```python
from build123d import *

# Parameters (mm, degrees)
BOSS_EXTRUDE1_DEPTH = 88.9
SKETCH2_R           = 3.175
CUT_EXTRUDE1_DEPTH  = 38.1
SKETCH3_R           = 4.1275
CUT_EXTRUDE2_DEPTH  = 25.4


with BuildPart() as part:
    # Sketch1 → Boss-Extrude1 (new body)
    with BuildSketch(Plane(origin=(0, 0, 0), x_dir=(1, 0, 0), z_dir=(0, 1, 0))):
        Polygon((0, 0), (38.1, 38.1), (76.2, 38.1), (76.2, 0), align=None)
    extrude(amount=BOSS_EXTRUDE1_DEPTH)

    # Sketch2 → Cut-Extrude1 (cut)
    with BuildSketch(Plane(origin=(38.1, 0, 38.1), x_dir=(-0.7071067811865464, 0, 0.7071067811865488), z_dir=(-0.7071067811865488, 0, -0.7071067811865464))):
        with Locations(Location((-28.481536726, 69.85, 0), (0, 0, 180))):
            Circle(SKETCH2_R)
        with Locations(Location((-29.901764766, 19.05, 0), (0, 0, 180))):
            Circle(SKETCH2_R)
    extrude(amount=CUT_EXTRUDE1_DEPTH, mode=Mode.SUBTRACT)

    # Sketch3 → Cut-Extrude2 (cut)
    with BuildSketch(Plane(origin=(76.2, 0, 0), x_dir=(0, 0, -1), z_dir=(1, 0, 0))):
        with Locations((19.05, 44.45)):
            Circle(SKETCH3_R)
    extrude(amount=-CUT_EXTRUDE2_DEPTH, mode=Mode.SUBTRACT)


solid = part.part
```
Work out the finished part from the listing and answer in its coordinate system (mm). A direction names the side the tool comes from. Give positions to 0.01 mm unless a question says otherwise; leave off trailing zeros. Write each loop counter-clockwise with the first axis right and the second up, starting at its lowest first coordinate (ties: lowest second). Pieces come first, ordered by that corner, then holes.
(1) The mould has two halves that part along Y. Classify faces 1 (the flat face through (31.27, 69.81, -8.95)), 2 (the flat face through (57, 44, -38.1)), 3 (the flat face through (47, 0, -19)): pulls with the +Y half, pulls with the -Y half, needs draft (parallel to the pull), parting line crosses it, or undercut.
Final values:
face 1: undercut
face 2: needs draft
face 3: pulls with the -Y half
(2) The part is cut by section D-D on x = 14. Write down the section's boundary in (y, z), plus the area to 3 significant figures.
Final values:
outline: (0, -14) - (88.9, -14) - (88.9, 0) - (0, 0) - close
area: 1,240 mm2
(3) Flat-ended cylindrical pins translate along their axes: pin 1 Ø2.5 at (y, z) = (45.5, -19) entering from +X; pin 2 Ø1.5 at (y, z) = (50, -20.5) entering from -X; pin 3 Ø3 at (y, z) = (39.5, -28.5) entering from -X. Find the tip coordinate at first contact, or state that the pin passes through.
Final values:
pin 1: stops at x = 50.8
pin 2: stops at x = 19.75
pin 3: stops at x = 27
(4) The part is cut by section B-B on z = -19.05. Write down the section's boundary in (x, y), plus the area to 3 significant figures.
Final values:
outline: (19.05, 0) - (76.2, 0) - (76.2, 40.32) - (50.8, 40.32) - (50.8, 48.58) - (76.2, 48.58) - (76.2, 88.9) - (19.05, 88.9) - close
area: 4,870 mm2
(5) The part is cut by section C-C on y = 44.45. Write down the section's boundary in (x, z).
Final values:
outline: (0, 0) - (38.1, -38.1) - (76.2, -38.1) - (76.2, -23.18) - (50.8, -23.18) - (50.8, -14.92) - (76.2, -14.92) - (76.2, 0) - close
(6) Which of the six approach directions +Z, -Z, +X, -X, +Y, -Y give full straight-line access (tool end or side, diameter ignored) to faces 4 (the flat face through (76.2, 44, -24)), 5 (the flat face through (32.27, 19.01, -9.95)), 6 (the cylindrical face through (63.678, 45.69, -22.987))?
Final values:
face 4: +Z, -Z, +X, +Y, -Y
face 5: none
face 6: +X
(7) Straight lines are drawn through the part: line 1 (Y direction, x = 64.5, z = -19.05); line 2 (Z direction, x = 66, y = 44); line 3 (X direction, y = 19, z = -9.5). For each, find the intervals that lie inside material, in ascending order.
Final values:
line 1: y = 0 to 40.32, 48.58 to 88.9
line 2: z = -38.1 to -23.15, -14.95 to 0
line 3: x = 9.5 to 31.82, 37.28 to 76.2
